```python
from build123d import *

# Parameters (mm, degrees)
ESBO_O1_R                                            = 6
EXTRUS_O1_DEPTH                                      = 36
ESBO_O2_R                                            = 10.5
EXTRUS_O2_DEPTH                                      = 2.2
ESBO_O3_R                                            = 10.5
EXTRUS_O3_DEPTH                                      = 2.2
ESBO_O4_R                                            = 1.65
EXTRUS_O4_DEPTH                                      = 26
ESCAREADO_PARA_PARAFUSO_DE_M_QUINA_COM_C_D           = 5.5
ESCAREADO_PARA_PARAFUSO_DE_M_QUINA_COM_C_DEPTH       = 12
ESCAREADO_PARA_PARAFUSO_DE_M_QUINA_COM_C_CSINK_D     = 9
ESCAREADO_PARA_PARAFUSO_DE_M_QUINA_COM_C_CSINK_ANGLE = 90
ESCAREADO_PARA_PARAFUSO_DE_M_QUINA_COM_C_TIP         = 1.652366702
ESCAREADO_PARA_SFHCS_M41_D                           = 4.5
ESCAREADO_PARA_SFHCS_M41_CSINK_D                     = 8.96
ESCAREADO_PARA_SFHCS_M41_CSINK_ANGLE                 = 90


with BuildPart() as part:
    # Esboço1 → Extrusão1 (new body)
    with BuildSketch(Plane.XY):
        with BuildLine():
            Line((-20, 10), (-20, -6))
            Line((-20, -6), (-21, -7))
            Line((-21, -7), (-21, -15))
            Line((-21, -15), (-9.5, -15))
            Line((-9.5, -15), (-8.5, -14))
            Line((-8.5, -14), (-3.5, -14))
            Line((-3.5, -14), (-2.5, -15))
            Line((-2.5, -15), (2.5, -15))
            Line((2.5, -15), (3.5, -14))
            Line((3.5, -14), (8.5, -14))
            Line((8.5, -14), (9.5, -15))
            Line((9.5, -15), (21, -15))
            Line((21, -15), (21, -7))
            Line((21, -7), (20, -6))
            Line((20, -6), (20, 10))
            Line((20, 10), (9.797958971, 10))
            ThreePointArc((9.797958971, 10), (0, 14), (-9.797958971, 10))
            Line((-9.797958971, 10), (-20, 10))
        make_face()
        Circle(ESBO_O1_R, mode=Mode.SUBTRACT)
    extrude(amount=EXTRUS_O1_DEPTH)

    # Esboço2 → Extrusão2 (cut)
    with BuildSketch(Plane.XY.offset(36)):
        Circle(ESBO_O2_R)
    extrude(amount=-EXTRUS_O2_DEPTH, mode=Mode.SUBTRACT)

    # Esboço3 → Extrusão3 (cut)
    with BuildSketch(Plane(origin=(0, 0, 0), x_dir=(-1, 0, 0), z_dir=(0, 0, -1))):
        Circle(ESBO_O3_R)
    extrude(amount=-EXTRUS_O3_DEPTH, mode=Mode.SUBTRACT)

    # Esboço4 → Extrusão4 (cut, through all)
    with BuildSketch(Plane(origin=(0, 10, 0), x_dir=(1, 0, 0), z_dir=(0, 1, 0))):
        with Locations((15.25, -5)):
            Circle(ESBO_O4_R)
        with Locations((15.25, -31)):
            Circle(ESBO_O4_R)
        with Locations((-15.25, -5)):
            Circle(ESBO_O4_R)
        with Locations((-15.25, -31)):
            Circle(ESBO_O4_R)
    extrude(amount=-EXTRUS_O4_DEPTH, mode=Mode.SUBTRACT)

    # Escareado para parafuso de máquina com cabeça chata de M52
    with Locations(Plane(origin=(-15.25, -15, 31), x_dir=(0, 0, -1), z_dir=(0, -1, 0))):
        with Locations((0, 0), (26, 0), (26, 30.5), (0, 30.5)):
            CounterSinkHole(ESCAREADO_PARA_PARAFUSO_DE_M_QUINA_COM_C_D / 2, ESCAREADO_PARA_PARAFUSO_DE_M_QUINA_COM_C_CSINK_D / 2, depth=ESCAREADO_PARA_PARAFUSO_DE_M_QUINA_COM_C_DEPTH, counter_sink_angle=ESCAREADO_PARA_PARAFUSO_DE_M_QUINA_COM_C_CSINK_ANGLE)
            with Locations((0, 0, -(ESCAREADO_PARA_PARAFUSO_DE_M_QUINA_COM_C_DEPTH + ESCAREADO_PARA_PARAFUSO_DE_M_QUINA_COM_C_TIP / 2))):  # 118° drill point
                Cone(0, ESCAREADO_PARA_PARAFUSO_DE_M_QUINA_COM_C_D / 2, ESCAREADO_PARA_PARAFUSO_DE_M_QUINA_COM_C_TIP, mode=Mode.SUBTRACT)

    # Escareado para SFHCS M41 (through all)
    with Locations(Plane(origin=(-15.25, 10, 5), x_dir=(0, 0, 1), z_dir=(0, 1, 0))):
        with Locations((0, 0), (26, 0), (26, 30.5), (0, 30.5)):
            CounterSinkHole(ESCAREADO_PARA_SFHCS_M41_D / 2, ESCAREADO_PARA_SFHCS_M41_CSINK_D / 2, counter_sink_angle=ESCAREADO_PARA_SFHCS_M41_CSINK_ANGLE)


solid = part.part
```
Read the model definition and answer for the solid it produces. Units are mm, in the model's axes. A direction names the side the tool comes from. Give positions to 0.01 mm unless a question says otherwise; leave off trailing zeros. Write each loop counter-clockwise with the first axis right and the second up, starting at its lowest first coordinate (ties: lowest second). Pieces come first, ordered by that corner, then holes. Notation, with made-up numbers: (19, -12) - (68, -12) arc R12 cw to (68, -1) - close; hole circle Ø1 at (-12.75, -26.75). An arc over 180 degrees is marked (long way). Write item = value, one per line. Start each with the question number.
Item 1: A tool of negligible diameter and unlimited length cuts with its end or side. For faces 1 (the cylindrical face through (15.371, -8.053, 28.253)), 2 (the flat face through (5, -5, 33.8)), 3 (the cylindrical face through (-10, 3.2, 1.1)), 4 (the flat face through (9, -14.5, 17.7)), from which of +Z, -Z, +X, -X, +Y, -Y can it reach the whole face along a straight path? Write none if from no direction.
Item 2: Find section C-C (z = 31). State how many separate pieces and enclosed holes the cut face has, then the cut area to 3 significant figures.
Item 3: The mould has two halves that part along Y. Classify faces 5 (the cylindrical face through (-14.42, -8.05, 7.62)), 6 (the cylindrical face through (-6, 0, 18)), 7 (the flat face through (-15, 10, 18)): +Y half, -Y half, draft (parallel to the pull), parting line (faces both ways), or undercut.
Item 4: Find section D-D (y = -7.5). Give the vertices of the cut face in (x, z), then the cut area to 3 significant figures.
Item 5: Find the intervals of material crossed by probe 1 along Z at (x, y) = (15.25, 1.5); probe 2 along Z at (x, y) = (15, -5); probe 3 along X at (y, z) = (1.5, 6), in increasing order. Write a range as [from, to].
Item 6: Each of these flat-tipped pins is pushed along its axis until it touches: P1, Ø5, axis at x = 16, z = 12.5, coming from the +Y side; P2, Ø12.5, axis at x = 0, y = 0, coming from the +Z side; P3, Ø6, axis at x = -4, z = 11.5, coming from the +Y side. Where does it stop, or does it pass through?
Item 7: Find section A-A (y = 0). Give the vertices of the cut face in (x, z), then the cut area to 3 significant figures.
Item 8: Find section B-B (x = -15.25). Give the vertices of the cut face in (y, z), then the cut area to 3 significant figures.
Response:
q1.face_1 = -Y
q1.face_2 = +Z
q1.face_3 = -Z
q1.face_4 = +Z, -Z, -Y
q2.separate_pieces = 3
q2.enclosed_holes = 1
q2.area = 680 mm²
q3.face_5 = draft
q3.face_6 = undercut
q3.face_7 = +Y half
q4.outline = (-21, 0) - (-7.35, 0) - (-7.35, 2.2) - (7.35, 2.2) - (7.35, 0) - (21, 0) - (21, 36) - (7.35, 36) - (7.35, 33.8) - (-7.35, 33.8) - (-7.35, 36) - (-21, 36) - close; hole circle Ø5.5 at (-15.25, 5); hole circle Ø5.5 at (-15.25, 31); hole circle Ø5.5 at (15.25, 5); hole circle Ø5.5 at (15.25, 31)
q4.area = 1,350 mm²
q5.probe_1 = [0, 2.75], [7.25, 28.75], [33.25, 36]
q5.probe_2 = [0, 2.26], [7.74, 28.26], [33.74, 36]
q5.probe_3 = [-20, -17.27], [-13.23, -5.81], [5.81, 13.23], [17.27, 20]
q6.P1 = 10
q6.P2 = 33.8
q6.P3 = 13.96
q7.outline = (-20, 0) - (-10.5, 0) - (-10.5, 2.2) - (-6, 2.2) - (-6, 33.8) - (-10.5, 33.8) - (-10.5, 36) - (-20, 36) - close; (6, 2.2) - (10.5, 2.2) - (10.5, 0) - (20, 0) - (20, 36) - (10.5, 36) - (10.5, 33.8) - (6, 33.8) - close; hole circle Ø4.5 at (-15.25, 5); hole circle Ø4.5 at (-15.25, 31); hole circle Ø4.5 at (15.25, 5); hole circle Ø4.5 at (15.25, 31)
q7.area = 905 mm²
q8.outline = (-15, 0) - (10, 0) - (10, 0.52) - (7.77, 2.75) - (-2.7, 2.75) - (-3, 2.25) - (-13.25, 2.25) - (-15, 0.5) - close; (-15, 9.5) - (-13.25, 7.75) - (-3, 7.75) - (-2.7, 7.25) - (7.77, 7.25) - (10, 9.48) - (10, 26.52) - (7.77, 28.75) - (-2.7, 28.75) - (-3, 28.25) - (-13.25, 28.25) - (-15, 26.5) - close; (-15, 35.5) - (-13.25, 33.75) - (-3, 33.75) - (-2.7, 33.25) - (7.77, 33.25) - (10, 35.48) - (10, 36) - (-15, 36) - close
q8.area = 635 mm²
